Read the model definition and answer for the solid it produces. Units are mm, in the model's axes. A direction names the side the tool comes from. Give positions to 0.01 mm unless a question says otherwise; leave off trailing zeros. Order: outer loops, then holes, each group sorted by start corner. A loop starts at its lowest first (then second) coordinate and runs counter-clockwise, first axis right, second up. Notation, with made-up numbers: (65.25, 9) - (79.25, 9) arc R28 cw to (79.25, 36) - close; hole circle Ø5 at (-2.75, 76). An arc over 180 degrees is marked (long way). Write each question's results on one line, items separated by ' | '.
from build123d import *

# Parameters (mm, degrees)
SKETCH091_W           = 44.5
SKETCH091_H           = 1.6
PAD034_DEPTH          = 6
POLARPATTERN017_COUNT = 24
HOLE001_D             = 4.5
HOLE001_DEPTH         = 25
HOLE001_CBORE_D       = 7
HOLE001_CBORE_DEPTH   = 4.4


with BuildPart() as part:
    # Sketch089 → Revolution011 (revolve)
    with BuildSketch(Plane.XZ):
        Polygon((0, 34), (36, 34), (36, 41.4), (43.2, 41.4), (43.2, 34), (44.2, 34), (48, 41.4), (48, 45), (44, 45), (43.2, 42), (0, 42), align=None)
    revolve(axis=Axis((0, 0, 0), (0, 0, 1)))

    # Sketch091 → Pad034 (new body)
    with BuildSketch(Plane(origin=(0, 0, 42), x_dir=(0.991445, 0.130526, 0), z_dir=(0, 0, 1))):
        with Locations((22.25, 0)):
            Rectangle(SKETCH091_W, SKETCH091_H)
    pad034 = extrude(amount=-PAD034_DEPTH)

    # PolarPattern017: Pad034 ×24 about axis
    polarpattern017_axis = Axis((0, 0, 42), (0, 0, 1))
    for i in range(1, POLARPATTERN017_COUNT):
        add(pad034.rotate(polarpattern017_axis, i * 360 / POLARPATTERN017_COUNT))

    # Hole001
    with Locations(Plane(origin=(0, 0, 42), x_dir=(-1, 0, 0), z_dir=(0, 0, 1))):
        with Locations((5, 0), (-5, 0)):
            CounterBoreHole(HOLE001_D / 2, HOLE001_CBORE_D / 2, HOLE001_CBORE_DEPTH, depth=HOLE001_DEPTH)


solid = part.part
(1) Section B-B (x = 0) is taken. Give the vertices of the cut face in (y, z).
Conclusion:
outline: (-48, 41.4) - (-44.2, 34) - (-43.2, 34) - (-43.2, 41.4) - (-36, 41.4) - (-36, 34) - (36, 34) - (36, 41.4) - (43.2, 41.4) - (43.2, 34) - (44.2, 34) - (48, 41.4) - (48, 45) - (44, 45) - (43.2, 42) - (-43.2, 42) - (-44, 45) - (-48, 45) - close
(2) Section A-A (y = 0) is taken. State how many separate pieces and enclosed holes the cut face has, plus the area to 3 significant figures.
Conclusion:
separate pieces: 3 | enclosed holes: 0 | area: 566 mm^2
(3) For faces 3 (the face through (-5.7, 2.3, 37.6)), 4 (the face through (34, 20, 41.4)), determine the directions among +Z, -Z, +X, -X, +Y, -Y from which every point of the face is accessible in a straight line to the end or side of a thin tool.
Conclusion:
face 3: +Z | face 4: -Z
(4) The mould has two halves that part along X. Classify faces 1 (the face through (-30.883, 24.706, 38.738)), 2 (the face through (4.37, -39.31, 38.74)): pulls with the +X half, pulls with the -X half, needs draft (parallel to the pull), parting line crosses it, or undercut.
Conclusion:
face 1: undercut | face 2: undercut
(5) Each of these flat-tipped pins is pushed along its axis until it touches: pin 1 (5.5 mm diameter, centred on x = -5.5, y = 1, fed in from +Z); pin 2 (4.5 mm diameter, centred on x = 14.5, y = 37, fed in from -Z); pin 3 (6 mm diameter, centred on y = -24, z = 36.5, fed in from -X). Where does it stop, or does it pass through?
Conclusion:
pin 1: z = 42 | pin 2: z = 36 | pin 3: x = -41.12
(6) Section C-C (z = 43.25) is taken. Give the vertices of the cut face in (x, y), plus the area to 3 significant figures.
Conclusion:
outline: circle Ø96 at (0, 0); hole circle Ø87.07 at (0, 0) | area: 1,280 mm^2
(7) Consider probe 1 along Y at (x, z) = (-23, 39.25); probe 2 along Y at (x, z) = (5, 35.65); probe 3 along X at (y, z) = (27, 40.5). Determine where each line is inside the solid, lowest interval first. Write a range as [from, to].
Conclusion:
probe 1: [-40.87, -36.57], [-31.29, -28.66], [-27.69, 27.69], [28.66, 31.29], [36.57, 40.87] | probe 2: [-44.77, -42.91], [-35.65, -2.25], [2.25, 35.65], [42.91, 44.77] | probe 3: [-39.13, -33.72], [-23.81, 23.81], [33.72, 39.13]
